from build123d import *

# Parameters (mm, degrees)
CYLINDER004_R     = 19
CYLINDER004_DEPTH = 15
CYLINDER003_R     = 20
CYLINDER003_DEPTH = 17


with BuildPart() as cylinder001:
    # Cylinder004 → Cylinder004 (new body)
    with BuildSketch(Plane.XY.offset(3)):
        Circle(CYLINDER004_R)
    extrude(amount=CYLINDER004_DEPTH)


with BuildPart() as obj1:
    # Cylinder003 → Cylinder003 (new body)
    with BuildSketch(Plane.XY):
        Circle(CYLINDER003_R)
    extrude(amount=CYLINDER003_DEPTH)

    # Cut003: cut Cylinder001
    add(cylinder001.part, mode=Mode.SUBTRACT)


with BuildPart() as obj1_1:
    # Cut003 placement: moved
    add(obj1.part.moved(Location((0, 0, -39))))


solid = obj1_1.part
Geometry check sheet. Reference: the model listing, model coordinates, mm. A direction names the side the tool comes from. Give positions to 0.01 mm unless a question says otherwise; leave off trailing zeros. Order: outer loops, then holes, each group sorted by start corner. A loop starts at its lowest first (then second) coordinate and runs counter-clockwise, first axis right, second up.
1. Sectioned sample at C-C (z = -35.25). Record the boundary of the cut face in (x, y), then the cut area to 3 significant figures.
Completed:
outline: circle Ø40 at (0, 0); hole circle Ø38 at (0, 0)
area: 123 mm2
2. Depth check by flat-ended pin: pin 1 (4 mm diameter, centred on y = 12, z = -35, fed in from -X); pin 2 (6 mm diameter, centred on x = 7, y = 9, fed in from +Z); pin 3 (1.5 mm diameter, centred on x = 10.5, z = -36.5, fed in from -Y). Enter the tip coordinate at first touch or a pass-through.
Completed:
pin 1: stops at x = -17.32
pin 2: stops at z = -36
pin 3: stops at y = -17.46
3. Draft check along X on faces 1 (the face through (-4.336, -19.524, -30.619)), 2 (the face through (18, -7, -22)), 3 (the face through (0, 0, -36)). Enter one of: pulls with the +X half, pulls with the -X half, needs draft (parallel to the pull), parting line crosses it, or undercut.
Completed:
face 1: parting line crosses it
face 2: needs draft
face 3: undercut
4. Sectioned sample at A-A (x = 0). Record the boundary of the cut face in (y, z), then the cut area to 3 significant figures.
Completed:
outline: (-20, -39) - (20, -39) - (20, -22) - (19, -22) - (19, -36) - (-19, -36) - (-19, -22) - (-20, -22) - close
area: 148 mm2
5. Scan lines: line 1 (Y direction, x = 0, z = -29.75); line 2 (Z direction, x = 9.5, y = -2); line 3 (X direction, y = 11.5, z = -22.25). Record each from-to range of solid material in increasing order.
Completed:
line 1: y = -20 to -19, 19 to 20
line 2: z = -39 to -36
line 3: x = -16.36 to -15.12, 15.12 to 16.36
6. Access from +Z, -Z, +X, -X, +Y, -Y to the whole of each face (thin tool, end or side, straight path). Record for faces 4 (the face through (0, 0, -39)), 5 (the face through (8.767, -16.856, -29.098)).
Completed:
face 4: -Z, +X, -X, +Y, -Y
face 5: +Z
